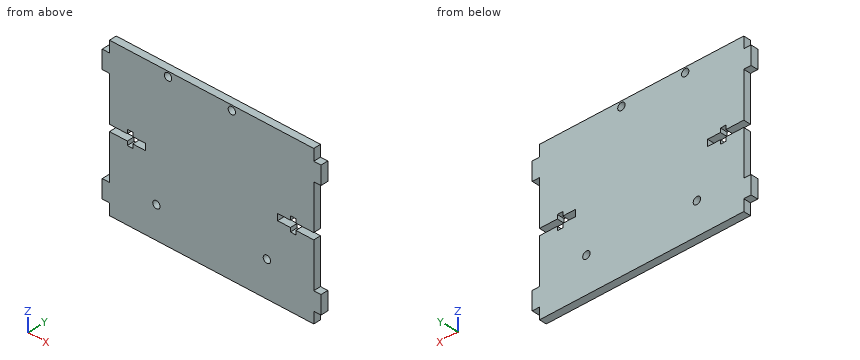
```python
from build123d import *

# Parameters (mm, degrees)
SKETCH1_R           = 1.6
BOSS_EXTRUDE1_DEPTH = 3.18
CUT_EXTRUDE1_DEPTH  = 71.077005804


with BuildPart() as part:
    # Sketch1 → Boss-Extrude1 (new body)
    with BuildSketch(Plane(origin=(0, 0, 0), x_dir=(1, 0, 0), z_dir=(0, 1, 0))):
        Polygon((44.64191244, 17.475260069), (-44.64191244, 17.475260069), (-44.64191244, 12.475260069), (-47.82191244, 12.475260069), (-47.82191244, 4.475260069), (-44.64191244, 4.475260069), (-44.64191244, -38.124739931), (-47.82191244, -38.124739931), (-47.82191244, -46.124739931), (-44.64191244, -46.124739931), (-44.64191244, -51.124739931), (44.64191244, -51.124739931), (44.64191244, -46.124739931), (47.82191244, -46.124739931), (47.82191244, -38.124739931), (44.64191244, -38.124739931), (44.64191244, 4.475260069), (47.82191244, 4.475260069), (47.82191244, 12.475260069), (44.64191244, 12.475260069), align=None)
        with Locations(Location((24.15, 1.875260069, 0), (0, 0, 90))):
            Circle(SKETCH1_R, mode=Mode.SUBTRACT)
        with Locations(Location((8.85, -48.924739931, 0), (0, 0, 90))):
            Circle(SKETCH1_R, mode=Mode.SUBTRACT)
        with Locations(Location((-19.05, -48.924739931, 0), (0, 0, 90))):
            Circle(SKETCH1_R, mode=Mode.SUBTRACT)
        with Locations(Location((-24.15, 3.475260069, 0), (0, 0, 90))):
            Circle(SKETCH1_R, mode=Mode.SUBTRACT)
    extrude(amount=BOSS_EXTRUDE1_DEPTH)

    # Sketch2 → Cut-Extrude1 (cut, through all)
    with BuildSketch(Plane(origin=(0, 3.18, 0), x_dir=(1, 0, 0), z_dir=(0, 1, 0))):
        Polygon((-44.64191244, -15.399739931), (-36.84191244, -15.399739931), (-36.84191244, -13.649739931), (-34.46191244, -13.649739931), (-34.46191244, -15.399739931), (-28.84191244, -15.399739931), (-28.84191244, -18.249739931), (-34.46191244, -18.249739931), (-34.46191244, -19.999739931), (-36.84191244, -19.999739931), (-36.84191244, -18.249739931), (-44.64191244, -18.249739931), align=None)
    cut_extrude1 = extrude(amount=-CUT_EXTRUDE1_DEPTH, mode=Mode.SUBTRACT)

    # Mirror1: Cut-Extrude1 across plane
    add(cut_extrude1.mirror(Plane(origin=(0, 0, 0), x_dir=(0, 0, 1), z_dir=(1, 0, 0))), mode=Mode.SUBTRACT)


solid = part.part
```
Design review of the part built by this model. Coordinates are the model's own, in mm. Coordinates: 2 decimals unless noted, no trailing zeros. Order: outer loops, then holes, each group sorted by start corner. A loop starts at its lowest first (then second) coordinate and runs counter-clockwise, first axis right, second up.
1) Take a section at B-B, the plane y = 2.05. State how many separate pieces and enclosed holes the cut face has, and give its area (3 significant figures).
2) Take a section at A-A, the plane x = 8.85. Give the boundary of the cut face in (y, z).
3) Clearance check with flat-ended pins moving along their axes: pin 1 (0.9 mm diameter, centred on y = 1.5, z = 19, fed in from +X); pin 2 (1 mm diameter, centred on y = 2.5, z = 5, fed in from -X); pin 3 (1.6 mm diameter, centred on x = -47, y = 1, fed in from +Z). State where each tip first meets the part, or that it passes through.
4) Wall thickness on line 1 along Z through (x, y) = (24.15, 0.8); line 2 along Z through (x, y) = (-36, 2.6); line 3 along X through (y, z) = (1.8, 48.5): over which ranges is each line inside the solid? List them lowest first.
Returned:
1. separate pieces: 1
1. enclosed holes: 4
1. area: 6,090 mm2
2. outline: (0, -17.48) - (3.18, -17.48) - (3.18, 47.32) - (0, 47.32) - close; (0, 50.52) - (3.18, 50.52) - (3.18, 51.12) - (0, 51.12) - close
3. pin 1: stops at x = 44.64
3. pin 2: stops at x = -44.64
3. pin 3: stops at z = 46.12
4. line 1: z = -17.48 to -3.48, -0.28 to 51.12
4. line 2: z = -17.48 to 13.65, 20 to 51.12
4. line 3: x = -44.64 to -20.59, -17.51 to 7.31, 10.39 to 44.64
